```python
from build123d import *

# Parameters (mm, degrees)
SKETCH1_R           = 22
BOSS_EXTRUDE1_DEPTH = 20


with BuildPart() as part:
    # Sketch1 → Boss-Extrude1 (new body)
    with BuildSketch(Plane.XY):
        with BuildLine():
            Line((-17.616288532, 0), (17.616288532, 0))
            ThreePointArc((17.616288532, 0), (22, -1.012059537), (25.496396068, -3.843385247))
            Line((25.496396068, -3.843385247), (52.5, -38.406422138))
            Line((52.5, -38.406422138), (58, -34.109351193))
            Line((58, -34.109351193), (96, -82.747133216))
            Line((96, -82.747133216), (96, -94.747133216))
            Line((96, -94.747133216), (-96, -94.747133216))
            Line((-96, -94.747133216), (-96, -82.747133216))
            Line((-96, -82.747133216), (-58, -34.109351193))
            Line((-58, -34.109351193), (-52.5, -38.406422138))
            Line((-52.5, -38.406422138), (-25.496396068, -3.843385247))
            ThreePointArc((-25.496396068, -3.843385247), (-22, -1.012059537), (-17.616288532, 0))
        make_face()
        with Locations((0, -32.247133216)):
            Circle(SKETCH1_R, mode=Mode.SUBTRACT)
    extrude(amount=BOSS_EXTRUDE1_DEPTH)

    # Cut-Sweep3: sweep along a path in Sketch2
    with BuildLine(Plane.XY.offset(20)) as cut_sweep3_path:
        Line((23.882346885, -13.588198867), (87.290655754, -94.747133216))
        Line((87.290655754, -94.747133216), (-87.290655754, -94.747133216))
        Line((-87.290655754, -94.747133216), (-23.882346885, -13.588198867))
        ThreePointArc((-23.882346885, -13.588198867), (0, -1.94), (23.882346885, -13.588198867))
    # Sketch3 → Cut-Sweep3 (sweep, cut)
    with BuildSketch(Plane(origin=(0, 0, 0), x_dir=(0, 0, -1), z_dir=(1, 0, 0))):
        Polygon((-20, -3.843385247), (-20, 31.059468925), (10, 31.059468925), align=None)
    sweep(path=cut_sweep3_path.line, transition=Transition.RIGHT, mode=Mode.SUBTRACT)


solid = part.part
```
Geometry: final body of the model. Coordinates: model frame, mm. A direction names the side the tool comes from. Round coordinates to 2 decimals unless told otherwise and drop trailing zeros. Order: outer loops, then holes, each group sorted by start corner. A loop starts at its lowest first (then second) coordinate and runs counter-clockwise, first axis right, second up. Notation, with made-up numbers: (41, 21.25) - (96, 21.25) arc R24 ccw to (96, 38.25) - close; hole circle Ø1 at (56, 83.25). An arc over 180 degrees is marked (long way). Write item = value, one per line. Start each with the question number.
Q1. Cut plane D-D on y = -65.5. Return the cut outline in (x, z).
Q2. Access query for faces 1 (the flat face through (-55.288, -36.228, 4.626)), 2 (the flat face through (1, -67, 20)). Directions: +Z, -Z, +X, -X, +Y, -Y. A direction counts if a zero-diameter tool reaches every point of the face in a straight line with its end or side. Return the directions, or none.
Q3. Cut plane A-A on x = 0. Return the cut outline in (y, z), and give its area (3 significant figures).
Q4. Cut plane C-C on x = -75.5. Return the cut outline in (y, z), and give its area (3 significant figures).
Q5. Pin query (flat end, axial travel): pin 1 (6 mm diameter, centred on y = -28, z = 10, fed in from +X); pin 2 (8 mm diameter, centred on x = -31.5, z = 16.5, fed in from +Y); pin 3 (12 mm diameter, centred on y = -37, z = 4.5, fed in from -X). Return the tip coordinate at first contact, or that it passes through.
Q6. Cut plane B-B on y = -29. Return the cut outline in (x, z), and give its area (3 significant figures).
Q7. Pull-direction query (X, two-part tool) for faces 3 (the cylindrical face through (21.943, -0.984, 6.325)), 4 (the cylindrical face through (-2.864, -10.434, 9.86)), 5 (the flat face through (55.21, -36.29, 4.63)), 6 (the cylindrical face through (-22.06, -1.04, 6.33)); classes: +X half, -X half, draft (parallel to the pull), parting line (faces both ways), or undercut.
Q8. Ray query, line 1 (Y direction, x = 0, z = 5.25); line 2 (X direction, y = -33.5, z = 6); line 3 (Y direction, x = 7, z = 11.25). Return the intervals inside material, ascending. Write a range as from..to.
Outcome:
q1.outline = (-82.53, 0) - (82.53, 0) - (82.53, 6.11) - (62.02, 20) - (-62.02, 20) - (-82.53, 6.11) - close
q2.face_1 = +Z, -Z, +Y
q2.face_2 = +Z, +X, -X, +Y, -Y
q3.outline = (-94.75, 0) - (-54.25, 0) - (-54.25, 20) - (-92.84, 20) - (-94.75, 18.36) - close; (-10.25, 0) - (0, 0) - (0, 16.7) - (-3.84, 20) - (-10.25, 20) - close
q3.area = 1,010 mm^2
q4.outline = (-94.75, 0) - (-56.51, 0) - (-56.51, 6.11) - (-82.75, 20) - (-92.84, 20) - (-94.75, 18.36) - close
q4.area = 581 mm^2
q5.pin_1 = 46.71
q5.pin_2 = -10.69
q5.pin_3 = -64.95
q6.outline = (-45.15, 0) - (-21.76, 0) - (-21.76, 20) - (-33.51, 20) - (-45.15, 12.11) - close; (21.76, 0) - (45.15, 0) - (45.15, 12.11) - (33.51, 20) - (21.76, 20) - close
q6.area = 844 mm^2
q7.face_3 = +X half
q7.face_4 = undercut
q7.face_5 = undercut
q7.face_6 = -X half
q8.line_1 = -94.75..-54.25, -10.25..0
q8.line_2 = -48.67..-21.96, 21.96..48.67
q8.line_3 = -94.75..-53.1, -11.39..0
